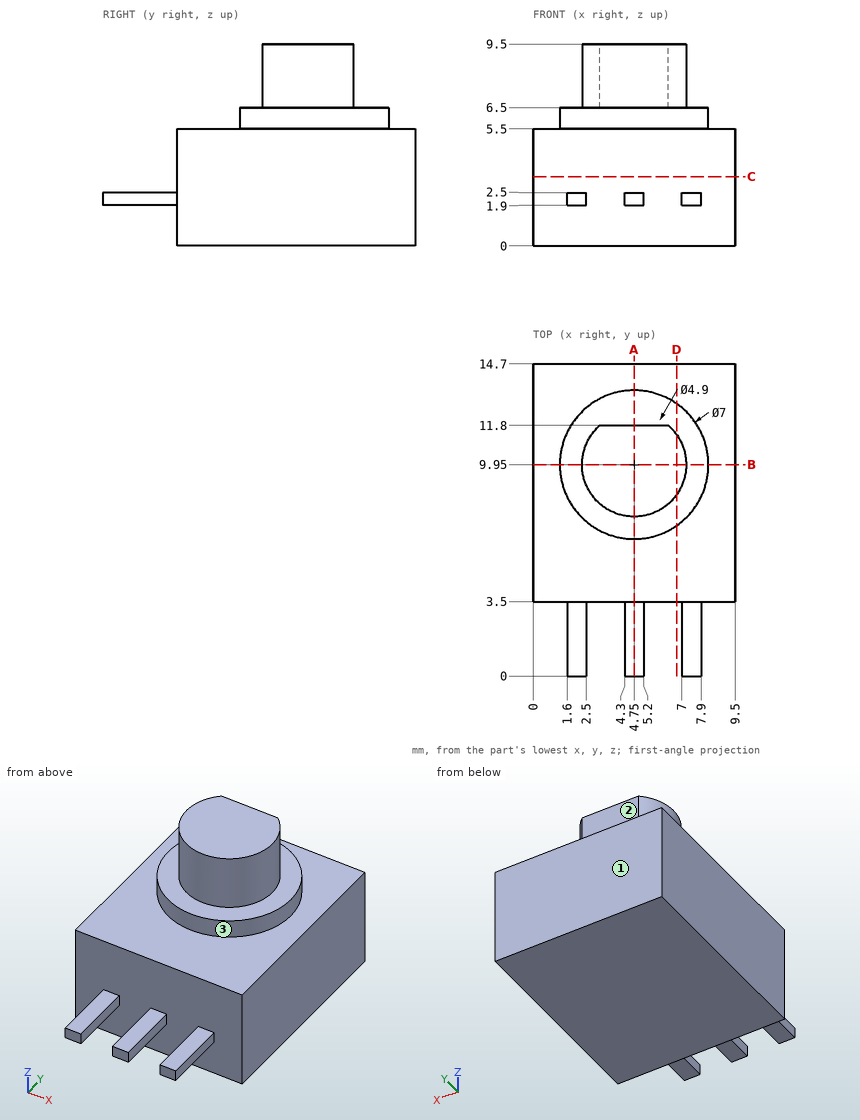
Input: dimensioned drawing with shaded views. Units: mm. Origin: part minimum x, y, z. A direction names the side the tool comes from. Give positions to 0.01 mm unless a question says otherwise; leave off trailing zeros. Loops run counter-clockwise (first coordinate to the right, second up) from the corner with the lowest first, then second, coordinate; pieces in that order, holes last. Notation, with made-up numbers: M 7,69 L 21,69 A17 cw 21,74 Z; hole C 81.5,-3 d3. An arc over 180 degrees is marked long. Put each result on its own line as item: value. Start each with the question number.
1) Cut plane D-D (x = 6.75). Output: boundary loops of the cut face in (y, z), then the cut area to 3 significant figures.
2) Contact query for flat-ended pins moving along their axis: pin 1 (0.5 mm diameter, centred on y = 1, z = 2, fed in from -X); pin 2 (1 mm diameter, centred on x = 7.5, y = 1.5, fed in from -Z); pin 3 (1 mm diameter, centred on x = 8.5, z = 8, fed in from +Y); pin 4 (2.5 mm diameter, centred on x = 5, z = 8, fed in from +Y). Output: stop coordinate, or through.
3) Access query for the marked faces 1, 2 and 3. Directions: +Z, -Z, +X, -X, +Y, -Y. A direction counts if a zero-diameter tool reaches every point of the face in a straight line with its end or side. Return the directions, or none.
4) Cut plane A-A (x = 4.75). Output: boundary loops of the cut face in (y, z), then the cut area to 3 significant figures.
5) Ray query, line 1 along Z through (x, y) = (7.5, 3.25); line 2 along Y through (x, z) = (6, 1.5); line 3 along Z through (x, y) = (7.5, 9.25). Return the intervals inside material, ascending.
6) Cut plane C-C (z = 3.25). Output: boundary loops of the cut face in (x, y), then the cut area to 3 significant figures.
7) Cut plane B-B (y = 9.95). Output: boundary loops of the cut face in (x, z), then the cut area to 4 significant figures.
Verdict:
1. outline: M 3.5,0 L 14.7,0 L 14.7,5.5 L 12.82,5.5 L 12.82,6.5 L 11.37,6.5 L 11.37,9.5 L 8.53,9.5 L 8.53,6.5 L 7.08,6.5 L 7.08,5.5 L 3.5,5.5 Z
1. area: 75.8 mm2
2. pin 1: x = 1.6
2. pin 2: z = 1.9
2. pin 3: through
2. pin 4: y = 11.8
3. face 1: +Z, -Z, +X, -X, +Y
3. face 2: +Z, +X, -X, +Y
3. face 3: +Z
4. outline: M 0,1.9 L 3.5,1.9 L 3.5,0 L 14.7,0 L 14.7,5.5 L 13.45,5.5 L 13.45,6.5 L 11.8,6.5 L 11.8,9.5 L 7.5,9.5 L 7.5,6.5 L 6.45,6.5 L 6.45,5.5 L 3.5,5.5 L 3.5,2.5 L 0,2.5 Z
4. area: 83.6 mm2
5. line 1: 1.9 to 2.5
5. line 2: 3.5 to 14.7
5. line 3: 0 to 6.5
6. outline: M 0,3.5 L 9.5,3.5 L 9.5,14.7 L 0,14.7 Z
6. area: 106 mm2
7. outline: M 0,0 L 9.5,0 L 9.5,5.5 L 8.25,5.5 L 8.25,6.5 L 7.2,6.5 L 7.2,9.5 L 2.3,9.5 L 2.3,6.5 L 1.25,6.5 L 1.25,5.5 L 0,5.5 Z
7. area: 73.95 mm2
